Source: CAD feature listing. Evaluate the final solid. Frame: model axes, mm. A direction names the side the tool comes from. Round coordinates to 2 decimals unless told otherwise and drop trailing zeros. Order: outer loops, then holes, each group sorted by start corner. A loop starts at its lowest first (then second) coordinate and runs counter-clockwise, first axis right, second up.
```python
from build123d import *

# Parameters (mm, degrees)
BOSS_EXTRUDE1_DEPTH = 0.5
SKETCH2_R           = 1.525
CUT_EXTRUDE1_DEPTH  = 0.5
BOSS_EXTRUDE2_DEPTH = 6.1
SKETCH9_R           = 1.825
SKETCH9_R_2         = 1.525
BOSS_EXTRUDE3_DEPTH = 0.5
SKETCH10_R          = 2.025
SKETCH10_R_2        = 1.525
BOSS_EXTRUDE4_DEPTH = 0.2
CUT_EXTRUDE2_DEPTH  = 6.6
FILLET1_R           = 0.4
FILLET2_R           = 0.4


with BuildPart() as part:
    # Sketch1 → Boss-Extrude1 (new body)
    with BuildSketch(Plane.XY):
        with BuildLine():
            Line((-14.42, 6.275), (14.42, 6.275))
            ThreePointArc((14.42, 6.275), (15.127106781, 5.982106781), (15.42, 5.275))
            Line((15.42, 5.275), (15.42, -5.275))
            ThreePointArc((15.42, -5.275), (15.127106781, -5.982106781), (14.42, -6.275))
            Line((14.42, -6.275), (-14.42, -6.275))
            ThreePointArc((-14.42, -6.275), (-15.127106781, -5.982106781), (-15.42, -5.275))
            Line((-15.42, -5.275), (-15.42, 5.275))
            ThreePointArc((-15.42, 5.275), (-15.127106781, 5.982106781), (-14.42, 6.275))
        make_face()
    extrude(amount=BOSS_EXTRUDE1_DEPTH)

    # Sketch2 → Cut-Extrude1 (cut)
    with BuildSketch(Plane.XY.offset(0.5)):
        with Locations((-12.495, 0)):
            Circle(SKETCH2_R)
        with Locations((12.495, 0)):
            Circle(SKETCH2_R)
    extrude(amount=-CUT_EXTRUDE1_DEPTH, mode=Mode.SUBTRACT)

    # Sketch3 → Boss-Extrude2 (add)
    with BuildSketch(Plane.XY.offset(0.5)):
        with BuildLine():
            Line((-6.00685473, 3.975), (6.00685473, 3.975))
            ThreePointArc((6.00685473, 3.975), (7.469056783, 3.339538441), (8.00208564, 1.836965157))
            Line((8.00208564, 1.836965157), (7.7288152, -2.113034843))
            ThreePointArc((7.7288152, -2.113034843), (7.098122731, -3.437202053), (5.73358429, -3.975))
            Line((5.73358429, -3.975), (-5.73358429, -3.975))
            ThreePointArc((-5.73358429, -3.975), (-7.098122731, -3.437202053), (-7.7288152, -2.113034843))
            Line((-7.7288152, -2.113034843), (-8.00208564, 1.836965157))
            ThreePointArc((-8.00208564, 1.836965157), (-7.469056783, 3.339538441), (-6.00685473, 3.975))
        make_face()
    extrude(amount=BOSS_EXTRUDE2_DEPTH)

    # Sketch9 → Boss-Extrude3 (add)
    with BuildSketch(Plane(origin=(0, 0, 0), x_dir=(-1, 0, 0), z_dir=(0, 0, -1))):
        with Locations((-12.495, 0)):
            Circle(SKETCH9_R)
        with Locations(Location((-12.495, 0, 0), (0, 0, 180))):
            Circle(SKETCH9_R_2, mode=Mode.SUBTRACT)
        with Locations((12.495, 0)):
            Circle(SKETCH9_R)
        with Locations(Location((12.495, 0, 0), (0, 0, 180))):
            Circle(SKETCH9_R_2, mode=Mode.SUBTRACT)
    extrude(amount=BOSS_EXTRUDE3_DEPTH)

    # Sketch10 → Boss-Extrude4 (add)
    with BuildSketch(Plane(origin=(0, 0, -0.5), x_dir=(-1, 0, 0), z_dir=(0, 0, -1))):
        with Locations((-12.495, 0)):
            Circle(SKETCH10_R)
        with Locations(Location((-12.495, 0, 0), (0, 0, 180))):
            Circle(SKETCH10_R_2, mode=Mode.SUBTRACT)
        with Locations((12.495, 0)):
            Circle(SKETCH10_R)
        with Locations(Location((12.495, 0, 0), (0, 0, 180))):
            Circle(SKETCH10_R_2, mode=Mode.SUBTRACT)
    extrude(amount=BOSS_EXTRUDE4_DEPTH)

    # Sketch11 → Cut-Extrude2 (cut)
    with BuildSketch(Plane.XY.offset(6.6)):
        with BuildLine():
            Line((-7.503277912, 1.871473868), (-7.230007472, -2.078526132))
            ThreePointArc((-7.230007472, -2.078526132), (-6.756988121, -3.071651539), (-5.73358429, -3.475))
            Line((-5.73358429, -3.475), (5.73358429, -3.475))
            ThreePointArc((5.73358429, -3.475), (6.756988121, -3.071651539), (7.230007472, -2.078526132))
            Line((7.230007472, -2.078526132), (7.503277912, 1.871473868))
            ThreePointArc((7.503277912, 1.871473868), (7.10350627, 2.998403831), (6.00685473, 3.475))
            Line((6.00685473, 3.475), (-6.00685473, 3.475))
            ThreePointArc((-6.00685473, 3.475), (-7.10350627, 2.998403831), (-7.503277912, 1.871473868))
        make_face()
    extrude(amount=-CUT_EXTRUDE2_DEPTH, mode=Mode.SUBTRACT)

    # Fillet1
    fillet1_edges = [part.edges().sort_by_distance(p)[0] for p in [
        (7.098122731, -3.437202053, 6.6),
        (7.86545042, -0.138034843, 6.6),
        (7.469056783, 3.339538441, 6.6),
        (0, 3.975, 6.6),
        (-7.469056783, 3.339538441, 6.6),
        (-7.86545042, -0.138034843, 6.6),
        (-7.098122731, -3.437202053, 6.6),
        (0, -3.975, 6.6),
    ]]
    fillet(fillet1_edges, radius=FILLET1_R)

    # Fillet2
    fillet2_edges = [part.edges().sort_by_distance(p)[0] for p in [
        (7.098122731, -3.437202053, 0.5),
        (7.86545042, -0.138034843, 0.5),
        (7.469056783, 3.339538441, 0.5),
        (0, 3.975, 0.5),
        (-7.469056783, 3.339538441, 0.5),
        (-7.86545042, -0.138034843, 0.5),
        (-7.098122731, -3.437202053, 0.5),
        (0, -3.975, 0.5),
    ]]
    fillet(fillet2_edges, radius=FILLET2_R)


solid = part.part
```
1. Pull-direction query (Y, two-part tool) for faces 4 (the face through (15.12, 5.99, 0.25)), 5 (the face through (0, -3.475, 3)), 6 (the face through (14.32, 0.08, -0.25)); classes: released by +Y, released by -Y, zero draft, split by the parting line, or undercut.
2. Access query for faces 1 (the face through (-10.67, 0.08, -0.25)), 2 (the face through (7.867, -0.11, 3.513)), 3 (the face through (-7.1, 3, 3.3)). Directions: +Z, -Z, +X, -X, +Y, -Y. A direction counts if a zero-diameter tool reaches every point of the face in a straight line with its end or side. Return the directions, or none.
3. Section A-A on z = 1.25. Return loops of the section in (x, y) (3 decimals), plus the area to 3 significant figures.
4. Section B-B on y = 0.5. State how many separate pieces and enclosed holes the cut face has, plus the area to 3 significant figures.
5. First-contact query: pin 1 (1.6 mm diameter, centred on x = -2.5, z = 2.5, fed in from -Y) (3 decimals); pin 2 (4 mm diameter, centred on y = -1, z = 4.5, fed in from -X); pin 3 (1.5 mm diameter, centred on y = -4, z = 2.5, fed in from -X). Flat tips, straight axial feed; report the tip coordinate or a pass-through.
6. Line query: line 1 along Y through (x, z) = (-5.5, 1) (3 decimals); line 2 along Z through (x, y) = (11, -3.75); line 3 along X through (y, z) = (-1.5, 3.25). Output: solid intervals per line, ascending.
Result:
1. face 4: released by +Y
1. face 5: undercut
1. face 6: split by the parting line
2. face 1: none
2. face 2: +Z, +X, -Y
2. face 3: +Z, -Z
3. outline: (-8.002, 1.837) - (-7.729, -2.113) arc R2 ccw to (-5.734, -3.975) - (5.734, -3.975) arc R2 ccw to (7.729, -2.113) - (8.002, 1.837) arc R2 ccw to (6.007, 3.975) - (-6.007, 3.975) arc R2 ccw to start; hole (-7.503, 1.871) - (-7.23, -2.079) arc R1.5 ccw to (-5.734, -3.475) - (5.734, -3.475) arc R1.5 ccw to (7.23, -2.079) - (7.503, 1.871) arc R1.5 ccw to (6.007, 3.475) - (-6.007, 3.475) arc R1.5 ccw to start
3. area: 21.2 mm2
4. separate pieces: 4
4. enclosed holes: 0
4. area: 12.3 mm2
5. pin 1: stops at y = -3.975
5. pin 2: stops at x = -7.94
5. pin 3: stops at x = -7.27
6. line 1: y = -3.975 to -3.475, 3.475 to 3.975
6. line 2: z = 0 to 0.5
6. line 3: x = -7.77 to -7.27, 7.27 to 7.77
